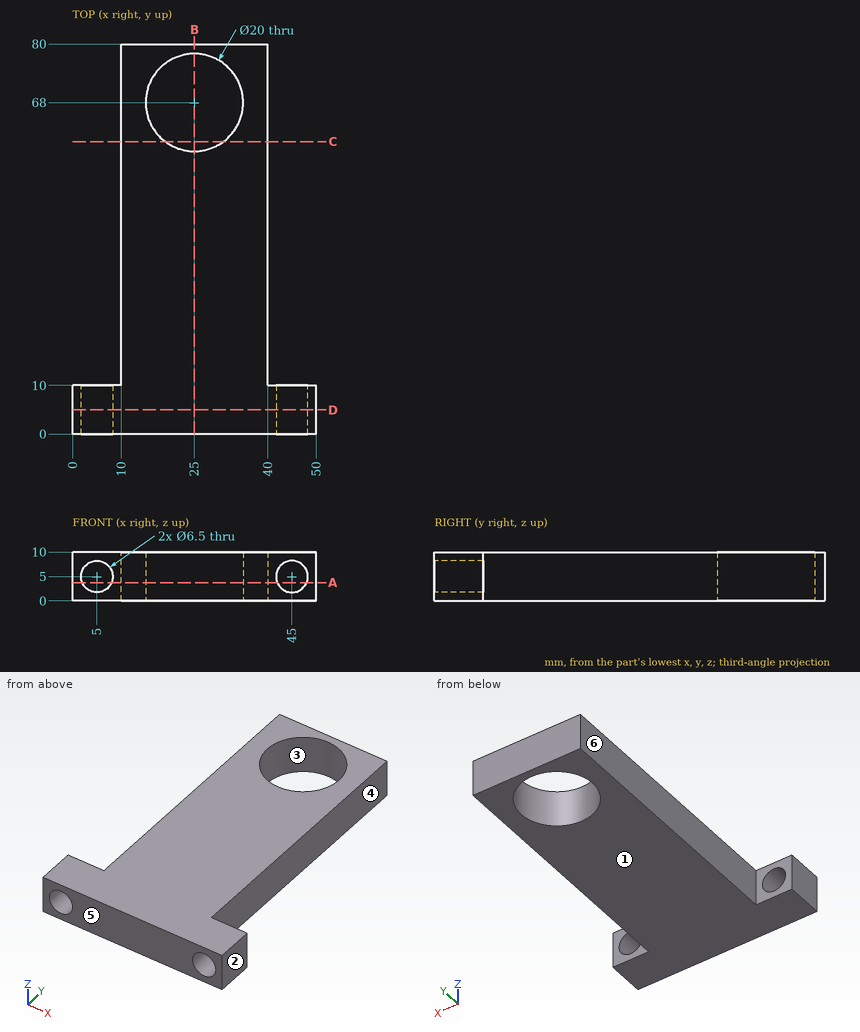
Input: dimensioned drawing with shaded views. Units: mm. Origin: part minimum x, y, z. A direction names the side the tool comes from. Coordinates: 2 decimals unless noted, no trailing zeros. Loops run counter-clockwise (first coordinate to the right, second up) from the corner with the lowest first, then second, coordinate; pieces in that order, holes last.
Q1. Section C-C, the plane y = 60. Return the cut outline in (x, z), and give its area (3 significant figures).
Results are:
outline: (10, 0) - (19, 0) - (19, 10) - (10, 10) - close; (31, 0) - (40, 0) - (40, 10) - (31, 10) - close
area: 180 mm2
Q2. Contact query for flat-ended pins moving along their axis: pin 1 (4 mm diameter, centred on x = 19, z = 2.5, fed in from -Y); pin 2 (5 mm diameter, centred on y = 52, z = 3, fed in from -X); pin 3 (3 mm diameter, centred on x = 3.5, z = 6.5, fed in from +Y). Output: stop coordinate, or through.
Results are:
pin 1: stops at y = 0
pin 2: stops at x = 10
pin 3: stops at y = 10
Q3. Set-up query: the marked faces 4, 5 and 6. Return all of +Z, -Z, +X, -X, +Y, -Y with unobstructed straight access to the full face (end or side cutting, diameter ignored); none if empty.
Results are:
face 4: +Z, -Z, +X, +Y
face 5: +Z, -Z, +X, -X, -Y
face 6: +Z, -Z, -X, +Y
Q4. Section D-D, the plane y = 5. Return the cut outline in (x, z), and give its area (3 significant figures).
Results are:
outline: (0, 0) - (50, 0) - (50, 10) - (0, 10) - close; hole circle Ø6.5 at (5, 5); hole circle Ø6.5 at (45, 5)
area: 434 mm2
Q5. Line query: line 1 along Z through (x, y) = (5, 3.25); line 2 along Y through (x, z) = (25, 2.25); line 3 along Y through (x, z) = (6, 8.5). Output: solid intervals per line, ascending.
Results are:
line 1: z = 0 to 1.75, 8.25 to 10
line 2: y = 0 to 58, 78 to 80
line 3: y = 0 to 10
Q6. Mould query, pull axis X, two halves, no side actions, for the marked faces 1, 2 and 3. Classes: +X half, -X half, draft (parallel to the pull), parting line (faces both ways), or undercut.
Results are:
face 1: draft
face 2: +X half
face 3: undercut
Q7. Section B-B, the plane x = 25. Return the cut outline in (y, z), and give its area (3 significant figures).
Results are:
outline: (0, 0) - (58, 0) - (58, 10) - (0, 10) - close; (78, 0) - (80, 0) - (80, 10) - (78, 10) - close
area: 600 mm2
Q8. Section A-A, the plane z = 3.75. Return the cut outline in (x, y), and give its area (3 significant figures).
Results are:
outline: (0, 0) - (2, 0) - (2, 10) - (0, 10) - close; (8, 0) - (42, 0) - (42, 10) - (40, 10) - (40, 80) - (10, 80) - (10, 10) - (8, 10) - close; (48, 0) - (50, 0) - (50, 10) - (48, 10) - close; hole circle Ø20 at (25, 68)
area: 2,170 mm2
